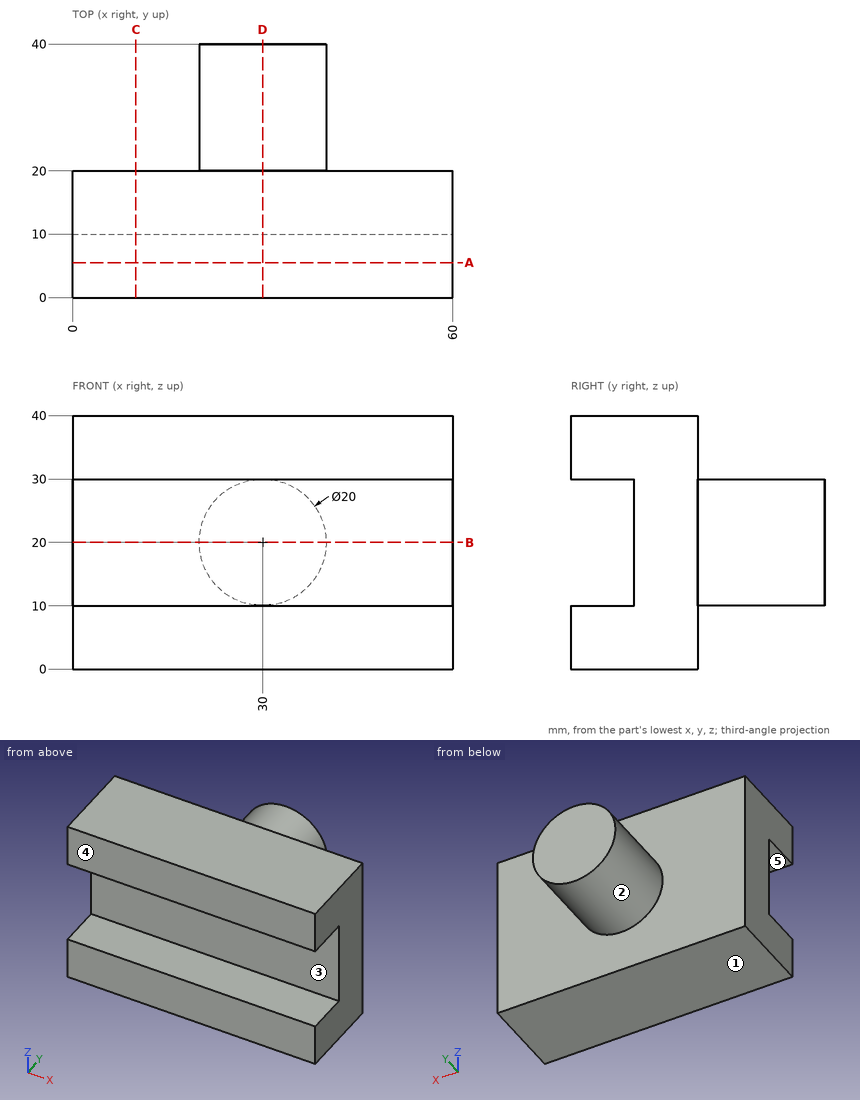
Print and shaded views of the part. All mm, measured from the part's lowest x, y and z. A direction names the side the tool comes from. Round coordinates to 2 decimals unless told otherwise and drop trailing zeros. Write each loop counter-clockwise with the first axis right and the second up, starting at its lowest first coordinate (ties: lowest second). Pieces come first, ordered by that corner, then holes.
Item 1: Two-plate mould, pull along Z, no slides. Class the marked faces 1, 2 and 3: +Z half, -Z half, draft (parallel to the pull), parting line (faces both ways), or undercut.
Results:
face 1: -Z half
face 2: parting line
face 3: undercut
Item 2: Cut at C-C, the plane x = 10. Give the cut face in (y, z), plus the area to 3 significant figures.
Results:
outline: (0, 0) - (20, 0) - (20, 40) - (0, 40) - (0, 30) - (10, 30) - (10, 10) - (0, 10) - close
area: 600 mm2
Item 3: Drop flat-ended pins along their axis: pin 1 Ø6 at (x, z) = (8, 32) entering from +Y; pin 2 Ø8 at (x, y) = (17.5, 17.5) entering from -Z; pin 3 Ø10 at (y, z) = (26.5, 15) entering from +X; pin 4 Ø1 at (x, z) = (53.5, 28) entering from -Y. Give the stop position or say it passes through.
Results:
pin 1: stops at y = 20
pin 2: stops at z = 0
pin 3: stops at x = 40
pin 4: stops at y = 10
Item 4: Which spindle directions (+Z, -Z, +X, -X, +Y, -Y) get a long thin tool onto all of the face, cutting with end or side? Do the marked faces 4 and 5. Say none if no direction does.
Results:
face 4: +Z, -Z, +X, -X, -Y
face 5: +X, -X, -Y
Item 5: Cut at B-B, the plane z = 20. Give the cut face in (x, y), plus the area to 3 significant figures.
Results:
outline: (0, 10) - (60, 10) - (60, 20) - (40, 20) - (40, 40) - (20, 40) - (20, 20) - (0, 20) - close
area: 1,000 mm2
Item 6: Cut at D-D, the plane x = 30. Give the cut face in (y, z).
Results:
outline: (0, 0) - (20, 0) - (20, 10) - (40, 10) - (40, 30) - (20, 30) - (20, 40) - (0, 40) - (0, 30) - (10, 30) - (10, 10) - (0, 10) - close
Item 7: Probe L1, parallel to Z at x = 39.5, y = 3.5; L2, parallel to Y at x = 28, z = 26.5; L3, parallel to Y at x = 16.5, z = 38.5. List the from-to ranges inside material, lowest first.
Results:
L1: z = 0 to 10, 30 to 40
L2: y = 10 to 40
L3: y = 0 to 20
Item 8: Cut at A-A, the plane y = 5.5. Give the cut face in (x, z), plus the area to 3 significant figures.
Results:
outline: (0, 0) - (60, 0) - (60, 10) - (0, 10) - close; (0, 30) - (60, 30) - (60, 40) - (0, 40) - close
area: 1,200 mm2
